Can you work these out from the drawing? Everything is in mm from the part's minimum corner. Coordinates: 2 decimals unless noted, no trailing zeros. Order: outer loops, then holes, each group sorted by start corner. A loop starts at its lowest first (then second) coordinate and runs counter-clockwise, first axis right, second up. Notation, with made-up numbers: (-24, 72) -> (17, 72) arc R15 ccw to (17, 84) -> close; hole circle Ø11 at (44.5, -12.5). An arc over 180 degrees is marked (long way). Answer in a Markdown table with one row per item.
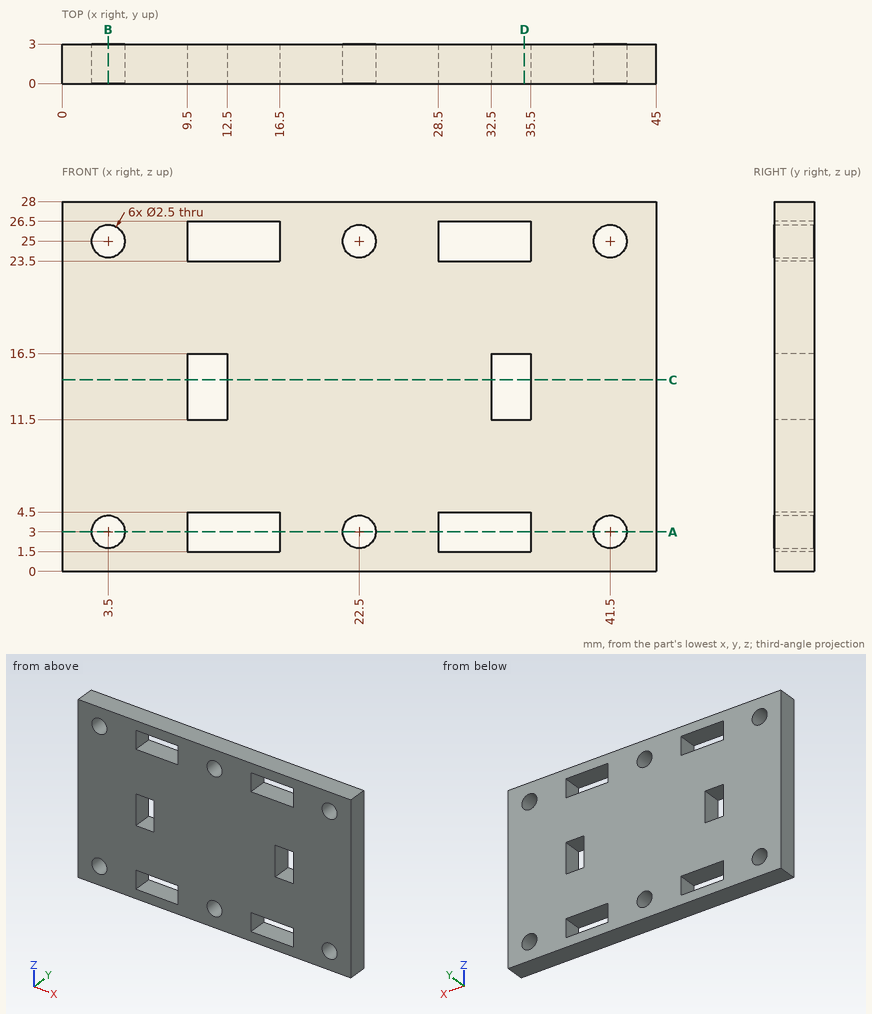
(1) Suppose I cut it at A-A (z = 3). Please give me the cut outline in (x, y), and give its area (3 significant figures).
Response values:
| item | result |
|---|---|
| outline | (0, 0) -> (2.25, 0) -> (2.25, 3) -> (0, 3) -> close; (4.75, 0) -> (9.5, 0) -> (9.5, 3) -> (4.75, 3) -> close; (16.5, 0) -> (21.25, 0) -> (21.25, 3) -> (16.5, 3) -> close; (23.75, 0) -> (28.5, 0) -> (28.5, 3) -> (23.75, 3) -> close; (35.5, 0) -> (40.25, 0) -> (40.25, 3) -> (35.5, 3) -> close; (42.75, 0) -> (45, 0) -> (45, 3) -> (42.75, 3) -> close |
| area | 70.5 mm2 |
(2) Suppose I cut it at D-D (x = 35). Please give me the cut outline in (y, z).
Response values:
| item | result |
|---|---|
| outline | (0, 0) -> (3, 0) -> (3, 1.5) -> (0, 1.5) -> close; (0, 4.5) -> (3, 4.5) -> (3, 11.5) -> (0, 11.5) -> close; (0, 16.5) -> (3, 16.5) -> (3, 23.5) -> (0, 23.5) -> close; (0, 26.5) -> (3, 26.5) -> (3, 28) -> (0, 28) -> close |
(3) Suppose I cut it at B-B (x = 3.5). Please give me the cut outline in (y, z).
Response values:
| item | result |
|---|---|
| outline | (0, 0) -> (3, 0) -> (3, 1.75) -> (0, 1.75) -> close; (0, 4.25) -> (3, 4.25) -> (3, 23.75) -> (0, 23.75) -> close; (0, 26.25) -> (3, 26.25) -> (3, 28) -> (0, 28) -> close |
(4) I need wall thicknesses on line 1 (Z direction, x = 22.5, y = 1.7); line 2 (Z direction, x = 33, y = 2.4); line 3 (X direction, y = 2.1, z = 25). Which ranges of each line are inside material? Lowest first, please. Write a range as [from, to].
Response values:
| item | result |
|---|---|
| line 1 | [0, 1.75], [4.25, 23.75], [26.25, 28] |
| line 2 | [0, 1.5], [4.5, 11.5], [16.5, 23.5], [26.5, 28] |
| line 3 | [0, 2.25], [4.75, 9.5], [16.5, 21.25], [23.75, 28.5], [35.5, 40.25], [42.75, 45] |
(5) Suppose I cut it at C-C (z = 14.5). Please give me the cut outline in (x, y).
Response values:
| item | result |
|---|---|
| outline | (0, 0) -> (9.5, 0) -> (9.5, 3) -> (0, 3) -> close; (12.5, 0) -> (32.5, 0) -> (32.5, 3) -> (12.5, 3) -> close; (35.5, 0) -> (45, 0) -> (45, 3) -> (35.5, 3) -> close |
